Job drawing, mm, ordinate dimensions from the low corner. One solid piece. A direction names the side the tool comes from. Coordinates: 2 decimals unless noted, no trailing zeros. Write each loop counter-clockwise with the first axis right and the second up, starting at its lowest first coordinate (ties: lowest second). Pieces come first, ordered by that corner, then holes. Notation, with made-up numbers: (24, 38.25) -> (59, 38.25) arc R16 ccw to (59, 60.25) -> close; hole circle Ø2 at (63, -21). An arc over 180 degrees is marked (long way). One line per question, with ' | ' between items. Start each with the question number.
Item 1: Saw through at B-B (z = 74.5). List the corners of the cut face in (x, y).
Item 2: Saw through at A-A (y = 241.3). List the corners of the cut face in (x, z) (3 decimals).
Item 3: Two-plate mould, pull along Z, no slides. Class the marked faces 4, 5 and 6: pulls with the +Z half, pulls with the -Z half, needs draft (parallel to the pull), parting line crosses it, or undercut.
Item 4: 3-axis set-ups, long thin cutter, end or side, ignore diameter. For the marked faces 1, 2 and 3: which of +Z, -Z, +X, -X, +Y, -Y reach the whole face in a straight line?
Item 5: Pin check, flat tips, straight feed: pin 1 (9.5 mm diameter, centred on x = 6, y = 153.5, fed in from +Z); pin 2 (3 mm diameter, centred on x = 3.5, z = 61, fed in from -Y); pin 3 (5.5 mm diameter, centred on x = 9, y = 66.5, fed in from -Z). Stop position of each tip, or through.
Item 6: Probe probe 1 along Z at (x, y) = (4.5, 241.3) (3 decimals); probe 2 along Y at (x, z) = (5.5, 27.5); probe 3 along Y at (x, z) = (14, 87). List the from-to ranges inside material, lowest first. Write a range as [from, to].
Item 7: Saw through at D-D (x = 13.5). List the corners of the cut face in (y, z) (3 decimals).
Item 8: Saw through at C-C (z = 54). List the corners of the cut face in (x, y).
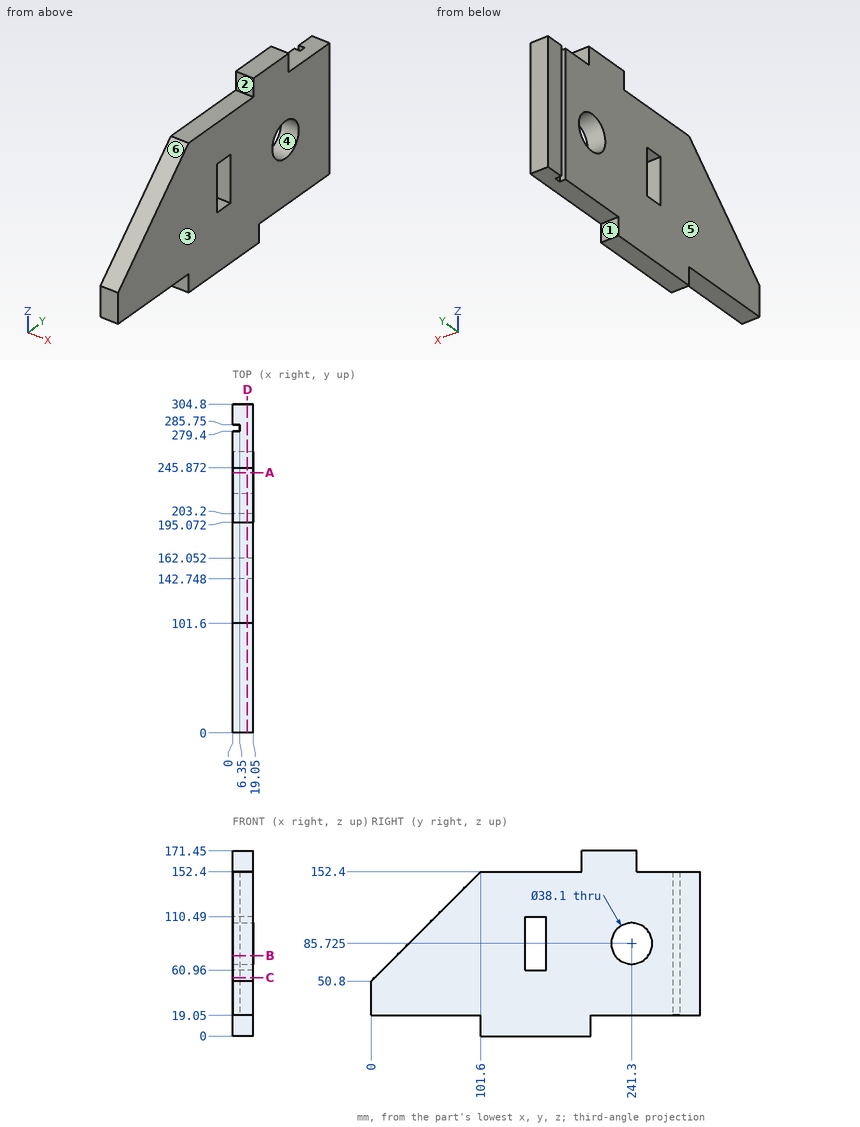
From the geometry:
1) outline: (0, 23.7) -> (19.05, 23.7) -> (19.05, 142.75) -> (0, 142.75) -> close; (0, 162.05) -> (19.05, 162.05) -> (19.05, 225.91) -> (0, 225.91) -> close; (0, 256.69) -> (19.05, 256.69) -> (19.05, 304.8) -> (0, 304.8) -> (0, 285.75) -> (6.35, 285.75) -> (6.35, 279.4) -> (0, 279.4) -> close
2) outline: (0, 19.05) -> (19.05, 19.05) -> (19.05, 66.675) -> (0, 66.675) -> close; (0, 104.775) -> (19.05, 104.775) -> (19.05, 171.45) -> (0, 171.45) -> close
3) face 4: undercut | face 5: needs draft | face 6: pulls with the +Z half
4) face 1: -Z, +X, -X, +Y | face 2: +Z, +X, -X, -Y | face 3: +Z, -Z, +X, +Y, -Y
5) pin 1: z = 152.4 | pin 2: y = 8.7 | pin 3: z = 19.05
6) probe 1: [19.05, 66.675], [104.775, 171.45] | probe 2: [0, 279.4], [285.75, 304.8] | probe 3: [36.2, 142.75], [162.05, 222.29], [260.31, 304.8]
7) outline: (0, 19.05) -> (101.6, 19.05) -> (101.6, 0) -> (203.2, 0) -> (203.2, 19.05) -> (304.8, 19.05) -> (304.8, 152.4) -> (245.872, 152.4) -> (245.872, 171.45) -> (195.072, 171.45) -> (195.072, 152.4) -> (101.6, 152.4) -> (0, 50.8) -> close; hole (142.748, 60.96) -> (162.052, 60.96) -> (162.052, 110.49) -> (142.748, 110.49) -> close; hole circle Ø38.1 at (241.3, 85.725)
8) outline: (0, 3.2) -> (19.05, 3.2) -> (19.05, 304.8) -> (0, 304.8) -> (0, 285.75) -> (6.35, 285.75) -> (6.35, 279.4) -> (0, 279.4) -> close
